Part model, mm, in its own coordinate system. A direction names the side the tool comes from. Round coordinates to 2 decimals unless told otherwise and drop trailing zeros. Loops run counter-clockwise (first coordinate to the right, second up) from the corner with the lowest first, then second, coordinate; pieces in that order, holes last. Notation, with made-up numbers: (62.5, 81) -> (106.5, 81) arc R27 cw to (106.5, 114) -> close; hole circle Ø3 at (0.5, 69). An arc over 180 degrees is marked (long way). Use a Markdown table: item, result. Add a question column.
Item 1: Which spindle directions (+Z, -Z, +X, -X, +Y, -Y) get a long thin tool onto all of the face, cutting with end or side? Do faces 1 (the face through (1, 9, 72)), 2 (the face through (3, 11, 66)), 3 (the face through (0.06, 3.04, 30.25)). Say none if no direction does.
Item 2: Cut at C-C, the plane z = 67.5. List the corners of the cut face in (x, y).
Item 3: Two-plate mould, pull along X, no slides. Class faces 4 (the face through (-27, 8, 83)), 5 (the face through (0, 3, -5)), 6 (the face through (-2.75, 3, 18)): pulls with the +X half, pulls with the -X half, needs draft (parallel to the pull), parting line crosses it, or undercut.
Item 4: Probe line 1 (X direction, y = 4.85, z = 35); line 2 (Z direction, x = 2.5, y = 4.75); line 3 (Y direction, x = -9, z = 27). List the from-to ranges inside material, lowest first. Write a range as [from, to].
Item 5: Flat gauge pins, fed straight in: pin 1 (17.5 mm diameter, centred on x = -14, z = 22, fed in from +Y); pin 2 (3.5 mm diameter, centred on y = 5, z = 34, fed in from -X); pin 3 (8 mm diameter, centred on x = -6, y = 8.5, fed in from -Z). Where does each tip first touch, or does it go through?
Item 6: Cut at D-D, the plane y = 13.25. List the corners of the cut face in (x, z).
Item 7: Cut at B-B, the plane y = 4.75. List the corners of the cut face in (x, z).
Item 8: Cut at A-A, the plane z = 35. List the corners of the cut face in (x, y), plus the area to 3 significant figures.
```python
from build123d import *

# Parameters (mm, degrees)
BOSS_EXTRUDE1_DEPTH             = 6
BOSS_EXTRUDE2_DEPTH             = 10
BOSS_EXTRUDE2_DIRECTION_2_REACH = 87.358
RIB1_REACH                      = 92.609
SKETCH3_WALL_W                  = 266.260300784
SKETCH3_WALL_H                  = 3
CUT_EXTRUDE1_REACH              = 91.744
SKETCH4_R                       = 1.75
BOSS_EXTRUDE3_DEPTH             = 4
CUT_EXTRUDE2_REACH              = 91.744


with BuildPart() as part:
    # Sketch1 → Boss-Extrude1 (new body)
    with BuildSketch(Plane(origin=(0, 0, 0), x_dir=(1, 0, 0), z_dir=(0, 1, 0))):
        with BuildLine():
            Line((5, 0), (5, -85))
            Line((5, -85), (-5, -85))
            Line((-5, -85), (-5, 0))
            ThreePointArc((-5, 0), (0, 5), (5, 0))
        make_face()
    extrude(amount=BOSS_EXTRUDE1_DEPTH)

    # Sketch2 → Boss-Extrude2 (add)
    with BuildSketch(Plane(origin=(0, 6, 0), x_dir=(1, 0, 0), z_dir=(0, 1, 0))):
        with BuildLine():
            Line((5, -81), (5, -85))
            Line((5, -85), (-25, -85))
            ThreePointArc((-25, -85), (-27, -83), (-25, -81))
            Line((-25, -81), (5, -81))
        make_face()
    extrude(amount=BOSS_EXTRUDE2_DEPTH)

    # Boss-Extrude2 direction 2: up to this face of the body (flat: up to its plane)
    boss_extrude2_direction_2_end = Plane(part.part.faces().sort_by_distance((0, 0, 40.529502163))[0])
    # Sketch2 → Boss-Extrude2 direction 2 (add, up to the picked face)
    with BuildSketch(Plane(origin=(0, 6, 0), x_dir=(1, 0, 0), z_dir=(0, 1, 0)), mode=Mode.PRIVATE) as boss_extrude2_direction_2_sk1:
        with BuildLine():
            Line((5, -81), (5, -85))
            Line((5, -85), (-25, -85))
            ThreePointArc((-25, -85), (-27, -83), (-25, -81))
            Line((-25, -81), (5, -81))
        make_face()
    boss_extrude2_direction_2_tool1 = split(extrude(boss_extrude2_direction_2_sk1.sketch, amount=-BOSS_EXTRUDE2_DIRECTION_2_REACH, mode=Mode.PRIVATE), bisect_by=boss_extrude2_direction_2_end, keep=Keep.BOTH, mode=Mode.PRIVATE)
    add(boss_extrude2_direction_2_tool1.solids().sort_by(Axis((-10.788554, 6, 83), (0, -1, 0)))[0])

    # Sketch3 wall → Rib1 (add, up to next)
    with BuildSketch(Plane(origin=(-13, 0, 40.256880935), x_dir=(-0.192673122493, 0, 0.98126299628), z_dir=(0.98126299628, 0, 0.192673122493)), mode=Mode.PRIVATE) as rib1_sk1:
        with Locations((0, -1.5)):
            Rectangle(SKETCH3_WALL_W, SKETCH3_WALL_H)
    rib1_tool1 = extrude(rib1_sk1.sketch, amount=RIB1_REACH, mode=Mode.PRIVATE) - part.part
    add(rib1_tool1.solids().sort_by_distance((-13, 0, 40.256880935))[0])

    # Sketch4 → Cut-Extrude1 (cut, up to next)
    with BuildSketch(Plane(origin=(0, 6, 0), x_dir=(1, 0, 0), z_dir=(0, 1, 0)), mode=Mode.PRIVATE) as cut_extrude1_sk1:
        with Locations(Location((0, 0, 0), (0, 0, 270))):
            Circle(SKETCH4_R)
    cut_extrude1_tool1 = extrude(cut_extrude1_sk1.sketch, amount=-CUT_EXTRUDE1_REACH, mode=Mode.PRIVATE) & part.part
    # Sketch4 → Cut-Extrude1 (cut, up to next)
    with BuildSketch(Plane(origin=(0, 6, 0), x_dir=(1, 0, 0), z_dir=(0, 1, 0)), mode=Mode.PRIVATE) as cut_extrude1_sk2:
        with Locations(Location((0, -35, 0), (0, 0, 270))):
            Circle(SKETCH4_R)
    cut_extrude1_tool2 = extrude(cut_extrude1_sk2.sketch, amount=-CUT_EXTRUDE1_REACH, mode=Mode.PRIVATE) & part.part
    # Sketch4 → Cut-Extrude1 (cut, up to next)
    with BuildSketch(Plane(origin=(0, 6, 0), x_dir=(1, 0, 0), z_dir=(0, 1, 0)), mode=Mode.PRIVATE) as cut_extrude1_sk3:
        with BuildLine():
            Line((2.75, -7.5), (2.75, -27.5))
            ThreePointArc((2.75, -27.5), (0, -30.25), (-2.75, -27.5))
            Line((-2.75, -27.5), (-2.75, -7.5))
            ThreePointArc((-2.75, -7.5), (0, -4.75), (2.75, -7.5))
        make_face()
    cut_extrude1_tool3 = extrude(cut_extrude1_sk3.sketch, amount=-CUT_EXTRUDE1_REACH, mode=Mode.PRIVATE) & part.part
    add(cut_extrude1_tool1.solids().sort_by_distance((0, 6, 0))[0], mode=Mode.SUBTRACT)
    add(cut_extrude1_tool2.solids().sort_by_distance((0, 6, 35))[0], mode=Mode.SUBTRACT)
    add(cut_extrude1_tool3.solids().sort_by_distance((0, 6, 17.5))[0], mode=Mode.SUBTRACT)

    # Sketch5 → Boss-Extrude3 (add)
    with BuildSketch(Plane(origin=(5, 0, 0), x_dir=(0, 0, -1), z_dir=(1, 0, 0))):
        Polygon((-81, 16), (-51, 6), (-81, 6), align=None)
    extrude(amount=-BOSS_EXTRUDE3_DEPTH)

    # Sketch6 → Cut-Extrude2 (cut, up to next)
    with BuildSketch(Plane(origin=(0, 6, 0), x_dir=(1, 0, 0), z_dir=(0, 1, 0)), mode=Mode.PRIVATE) as cut_extrude2_sk1:
        with BuildLine():
            Line((5, -40), (5, -46))
            ThreePointArc((5, -46), (2, -43), (5, -40))
        make_face()
    cut_extrude2_tool1 = extrude(cut_extrude2_sk1.sketch, amount=-CUT_EXTRUDE2_REACH, mode=Mode.PRIVATE) & part.part
    add(cut_extrude2_tool1.solids().sort_by_distance((3.72676, 6, 43))[0], mode=Mode.SUBTRACT)


solid = part.part
```
A:
| question | item | result |
|---|---|---|
| 1 | face 1 | -Z, -X, +Y |
| 1 | face 2 | -Z, +X, -X, +Y |
| 1 | face 3 | +Y, -Y |
| 2 | outline | (-18.35, 0) -> (5, 0) -> (5, 11.5) -> (1, 11.5) -> (1, 6) -> (-5, 6) -> (-5, 3) -> (-18.35, 3) -> close |
| 3 | face 4 | pulls with the -X half |
| 3 | face 5 | parting line crosses it |
| 3 | face 6 | undercut |
| 4 | line 1 | x = [-5, -1.75], [1.75, 5] |
| 4 | line 2 | z = [-4.33, 6.35], [28.65, 41.34], [44.66, 85] |
| 4 | line 3 | y = [0, 3] |
| 5 | pin 1 | stops at y = 3 |
| 5 | pin 2 | stops at x = -5 |
| 5 | pin 3 | stops at z = -4.09 |
| 6 | outline | (-25, 81) -> (1, 81) -> (1, 72.75) -> (5, 72.75) -> (5, 85) -> (-25, 85) arc R2 ccw to start |
| 7 | outline | (-25, 81) -> (-5, 81) -> (-5, 0) arc R5 ccw to (5, 0) -> (5, 40) arc R3 cw to (5, 46) -> (5, 85) -> (-25, 85) arc R2 ccw to start; hole (-2.75, 7.5) arc R2.75 ccw to (2.75, 7.5) -> (2.75, 27.5) arc R2.75 ccw to (-2.75, 27.5) -> close; hole circle Ø3.5 at (0, 0); hole circle Ø3.5 at (0, 35) |
| 8 | outline | (-11.97, 0) -> (-1.75, 0) -> (-1.75, 6) -> (-5, 6) -> (-5, 3) -> (-11.97, 3) -> close; (1.75, 0) -> (5, 0) -> (5, 6) -> (1.75, 6) -> close |
| 8 | area | 59.9 mm^2 |
